Job drawing, mm, ordinate dimensions from the low corner. One solid piece. A direction names the side the tool comes from. Give positions to 0.01 mm unless a question says otherwise; leave off trailing zeros. Write each loop counter-clockwise with the first axis right and the second up, starting at its lowest first coordinate (ties: lowest second). Pieces come first, ordered by that corner, then holes. Notation, with made-up numbers: (77, 87) - (117, 87) arc R25 cw to (117, 116) - close; hole circle Ø4 at (38.25, 71.5). An arc over 180 degrees is marked (long way). Use a Markdown table: item, result. Add a question column.
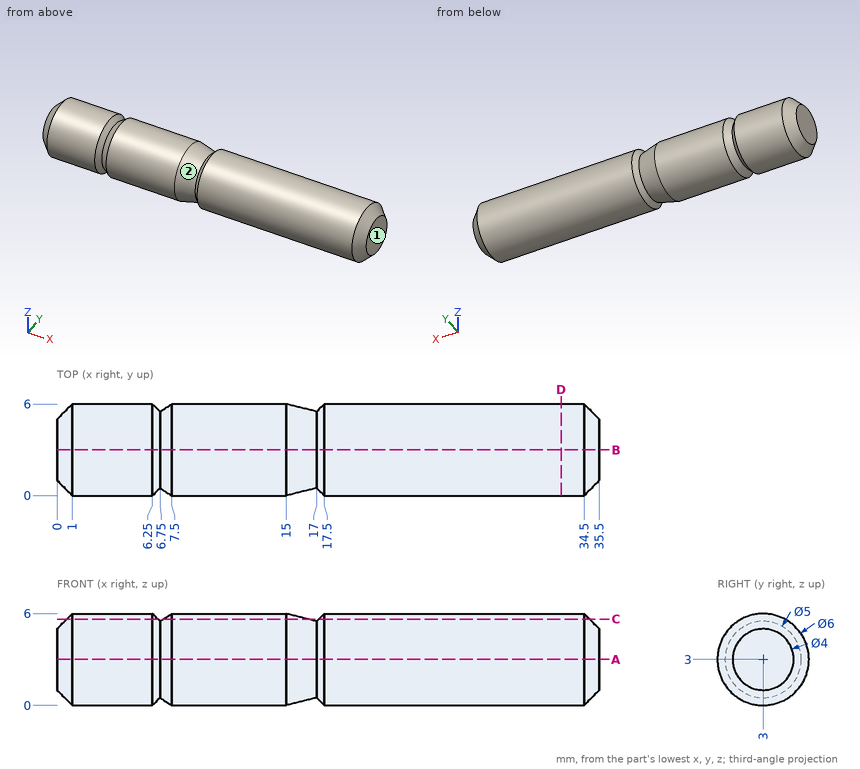
(1) Band-saw the part on D-D (x = 33). Write the cut outline in (y, z).
(2) Probe probe 1 along Y at (x, z) = (27, 3.1); probe 2 along Z at (x, y) = (16, 4.2); probe 3 along X at (y, z) = (1.8, 1.3). List the from-to ranges inside material, lowest first. Write a range as [from, to].
(3) Band-saw the part on C-C (z = 5.65). Give the number of separate pieces and of enclosed holes in the cut face, then the cut area to 3 significant figures.
(4) Which spindle directions (+Z, -Z, +X, -X, +Y, -Y) get a long thin tool onto all of the face, cutting with end or side? Do the marked faces 1 and 2. Say none if no direction does.
(5) Band-saw the part on A-A (z = 3). Write the cut outline in (x, y), then the cut area to 3 significant figures.
Model answer:
| question | item | result |
|---|---|---|
| 1 | outline | circle Ø6 at (3, 3) |
| 2 | probe 1 | y = [0, 6] |
| 2 | probe 2 | z = [0.53, 5.47] |
| 2 | probe 3 | x = [0.08, 35.42] |
| 3 | separate pieces | 3 |
| 3 | enclosed holes | 0 |
| 3 | area | 89.8 mm^2 |
| 4 | face 1 | +Z, -Z, +X, +Y, -Y |
| 4 | face 2 | none |
| 5 | outline | (0, 1) - (1, 0) - (6.25, 0) - (6.75, 0.5) - (7.5, 0) - (15, 0) - (17, 0.5) - (17.5, 0) - (34.5, 0) - (35.5, 1) - (35.5, 5) - (34.5, 6) - (17.5, 6) - (17, 5.5) - (15, 6) - (7.5, 6) - (6.75, 5.5) - (6.25, 6) - (1, 6) - (0, 5) - close |
| 5 | area | 209 mm^2 |
